```python
from build123d import *

# Parameters (mm, degrees)
F2_SIZE  = 5
F3_SIZE  = 5
F4_SIZE  = 3
F7_DEPTH = 32
F9_DEPTH = 5


with BuildPart() as f1:
    # F0 (on Front) → F1 (revolve)
    with BuildSketch(Plane.XZ):
        Polygon((-232.2130019963, 17.678354606), (-232.2130019963, -12.321645394), (252.7869980037, -12.321645394), (252.1408498287, 22.3974585533), (171.2869980037, 22.3974585533), (171.2869980037, 30.5355489254), (111.2869980037, 30.5355489254), (111.2869980037, 23.4147198498), (109.2869980037, 23.4147198498), (109.2869980037, 30.5355489254), (78.2869980037, 30.5355489254), (78.2869980037, 39.1822680831), (-16.7130019963, 39.1822680831), (-16.7130019963, 61.5620166063), (-36.7130019963, 61.5620166063), (-36.7130019963, 49.3548810482), (-91.7130019963, 49.3548810482), (-91.7130019963, 38.6736355722), (-139.7130019963, 38.6736355722), (-139.7130019963, 29.0096569806), (-191.2130019963, 29.0096569806), (-191.2130019963, 17.678354606), align=None)
    revolve(axis=Axis((10.0326761603, 0, -17.275730148), (1, 0, 0)))

    # F2
    f2_edges = [f1.edges().sort_by_distance(p)[0] for p in [
        (-232.213002, 0, -52.229815),
    ]]
    chamfer(f2_edges, length=F2_SIZE)

    # F3
    f3_edges = [f1.edges().sort_by_distance(p)[0] for p in [
        (252.14085, 0, -56.948919),
    ]]
    chamfer(f3_edges, length=F3_SIZE)

    # F4
    f4_edges = [f1.edges().sort_by_distance(p)[0] for p in [
        (-139.713002, 0, -73.225096),
    ]]
    chamfer(f4_edges, length=F4_SIZE)

    # F6 (on offset) → F7 (cut)
    with BuildSketch(Plane.XY.offset(50)):
        with BuildLine():
            Line((233.2867880477, 7.4999999971), (186.4272663162, 7.4986882053))
            ThreePointArc((186.4272663162, 7.4986882053), (178.8117069281, -0.608295434), (187.6377915852, -7.3773543158))
            Line((187.6377915852, -7.3773543158), (231.9362044222, -7.3773543158))
            Line((231.9362044222, -7.3773543158), (234.6377915852, -7.3773543158))
            ThreePointArc((234.6377915852, -7.3773543158), (240.7562641571, 0.6782795371), (233.2867880477, 7.4999999971))
        make_face()
    extrude(amount=-F7_DEPTH, mode=Mode.SUBTRACT)

    # F8 (on offset) → F9 (cut)
    with BuildSketch(Plane.XY.offset(50)):
        with BuildLine():
            Line((-76.4573437408, -7.4956413239), (-51.7143231445, -7.4999998836))
            ThreePointArc((-51.7143231445, -7.4999998836), (-44.2130030543, 0.003983777), (-51.7222906966, 7.499994248))
            Line((-51.7222906966, 7.499994248), (-76.0414618998, 7.4698750926))
            Line((-76.0414618998, 7.4698750926), (-77.4030428, 7.4681887824))
            ThreePointArc((-77.4030428, 7.4681887824), (-84.1980687904, -0.4730487165), (-76.4573437408, -7.4956413239))
        make_face()
    extrude(amount=-F9_DEPTH, mode=Mode.SUBTRACT)


solid = f1.part
```
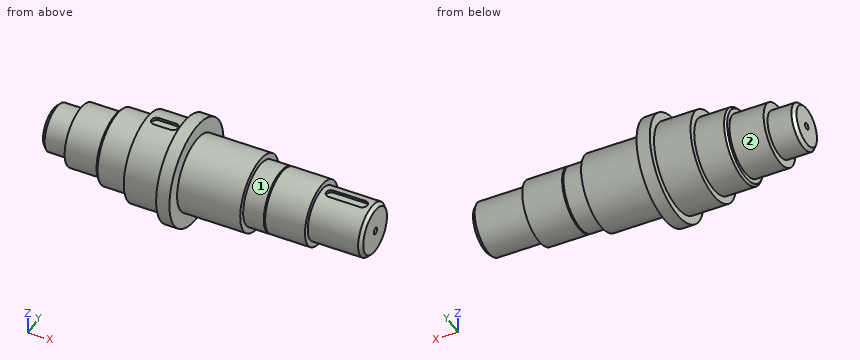
Here's how the part is built. I have some questions about the finished solid (model axes, mm). Face numbers are marked on the shaded views. A direction names the side the tool comes from. Give positions to 0.01 mm unless a question says otherwise; leave off trailing zeros. Write each loop counter-clockwise with the first axis right and the second up, starting at its lowest first coordinate (ties: lowest second). Pieces come first, ordered by that corner, then holes. Notation, with made-up numbers: (51.25, 40.5) -> (84.25, 40.5) arc R36 ccw to (84.25, 74.5) -> close; hole circle Ø9 at (5.5, 64.5). An arc over 180 degrees is marked (long way). Use one line per item in the form item = value.
1) On a 3-axis mill with a long thin cutter (end or side, diameter ignored), from which of +Z, -Z, +X, -X, +Y, -Y can I reach the whole of each face in a straight line? I mean the marked faces 1 and 2. Say none if no direction works.
Verdict:
face_1 = +X
face_2 = -X
2) Suppose I cut it at B-B (x = -99.5). Please give me the cut outline in (y, z).
Verdict:
outline = circle Ø111.9 at (0, -17.28); hole circle Ø9.91 at (0, -17.28)
3) I'm going to push flat-ended pins straight in: pin 1 (1.5 mm diameter, centred on x = 118.5, z = -36, fed in from -Y); pin 2 (5 mm diameter, centred on x = 18.5, y = -37.5, fed in from +Z); pin 3 (8 mm diameter, centred on x = 177.5, z = -6.5, fed in from -Y). Where does each tip first touch, or does it pass through?
Verdict:
pin_1 = -44.3
pin_2 = 27.02
pin_3 = -39.09
4) Suppose I cut it at A-A (x = 125.5). Please give me the cut outline in (y, z).
Verdict:
outline = circle Ø95.62 at (0, -17.28); hole circle Ø9.91 at (0, -17.28)
5) Suppose I cut it at C-C (x = 207). Please give me the cut outline in (y, z).
Verdict:
outline = (-7.38, 18) -> (-7.38, 21.71) arc R39.67 ccw (long way) to (7.5, 21.68) -> (7.5, 18) -> close; hole circle Ø9.91 at (0, -17.28)
6) If I drill on L1, parallel to Z at x = 82, y = 0; L2, parallel to Z at x = 11, y = 0; L3, parallel to Z at x = -101.5, y = 31.5, over which ranges is the centre line in solid material (lowest first)? Write a range as [from, to].
Verdict:
L1 = [-65.09, -22.23], [-12.32, 30.54]
L2 = [-73.73, -22.23], [-12.32, 39.18]
L3 = [-63.52, 28.96]
